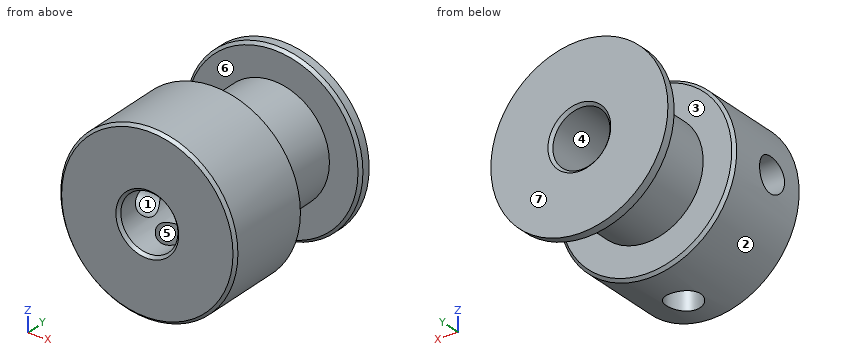
Autodesk Inventor part; units mm, degrees
ref_plane "YZ Plane" through (0, 0, 0) normal (1, 0, 0) x (0, 1, 0)
ref_plane "XZ Plane" through (0, 0, 0) normal (0, 1, 0) x (-1, 0, 0)
ref_plane "XY Plane" through (0, 0, 0) normal (0, 0, 1) x (1, 0, 0)
sketch "Эскиз1" plane through (0, 0, 0) normal (0, 1, 0) x (-1, 0, 0)
  circle A0 centre (0, 0) radius 7.75
  dimension "d0" = 15.5
extrude "Выдавливание1" add sketch "Эскиз1" along normal blind 8
sketch "Эскиз2" plane through (0, 8, 0) normal (0, 1, 0) x (1, 0, 0)
  circle A0 centre (0, 0) radius 5
  dimension "d3" = 10
extrude "Выдавливание2" add sketch "Эскиз2" along normal blind 7
sketch "Эскиз3" plane through (0, 15, 0) normal (0, 1, 0) x (1, 0, 0)
  circle A0 centre (0, 0) radius 7.75
extrude "Выдавливание3" add sketch "Эскиз3" along normal blind 1
chamfer "Фаска1" distance 0.25 angle 45 3 edges at (-7.75, 15, 0) (7.75, 8, 0) (7.75, 0, 0)
sketch "Эскиз4" plane through (0, 0, 0) normal (0, -1, 0) x (1, 0, 0)
  circle A0 centre (0, 0) radius 2.5
  dimension "d11" = 5
extrude "Выдавливание4" cut sketch "Эскиз4" against normal through all
chamfer "Фаска2" distance 0.25 angle 45 2 edges at (-2.5, 16, 0) (-2.5, 0, 0)
sketch "Эскиз5" plane through (0, 0, 0) normal (1, 0, 0) x (0, 1, 0)
  circle A0 centre (3.5, 0) radius 1.5
  point P0 (0, 0)
  dimension "d18" = 3
extrude "Выдавливание5" cut sketch "Эскиз5" against normal through all
sketch "Эскиз6" plane through (0, 0, 0) normal (0, 0, 1) x (1, 0, 0)
  circle A0 centre (0, 3.5) radius 1.5
  point P0 (0, 0)
  dimension "d22" = 3
extrude "Выдавливание6" cut sketch "Эскиз6" against normal through all
properties part number "GT2-20t"
Can you work these out from the model? Positions are in its coordinate system, mm. Face numbers are marked on the shaded views. A direction names the side the tool comes from. Coordinates: 2 decimals unless noted, no trailing zeros. Loops run counter-clockwise (first coordinate to the right, second up) from the corner with the lowest first, then second, coordinate; pieces in that order, holes last. Notation, with made-up numbers: (-29.75, 65) - (-6.75, 65) arc R36 ccw to (-6.75, 101) - close; hole circle Ø6 at (-14.75, 64). An arc over 180 degrees is marked (long way). Answer as a JSON object with one key per item and string values. Group by question number.
Item 1: If we mould it in two halves opening along Z, with no side actions, what happens to the marked faces 1, 2, 3 and 4? For each: released by +Z, released by -Z, zero draft, split by the parting line, or undercut.
Item 2: On a 3-axis mill with a long thin cutter (end or side, diameter ignored), from which of +Z, -Z, +X, -X, +Y, -Y can I reach the whole of each face in a straight line? I mean the marked faces 5, 6 and 7. Say none if no direction works.
Item 3: If I drill on L1, parallel to X at y = 12.5, z = 0; L2, parallel to Y at x = -3.5, z = 4.5; L3, parallel to Y at x = -6, z = -1.25, over which ranges is the centre line in solid material (lowest first)? Write a range as from..to.
Item 4: If we section it at D-D (y = 14.75): List the corners of the cut face in (x, z) for me, plus the area to 3 significant figures.
Item 5: If we section it at B-B (y = 4.5): List the corners of the cut face in (x, z) for me, plus the area to 3 significant figures.
Item 6: For pin 1 (4 mm diameter, centred on y = 10.5, z = -3, fed in from +X); pin 2 (1.8 mm diameter, centred on x = 0, y = 3.5, fed in from -Z); pin 3 (2 mm diameter, centred on x = -1, y = 13.5, fed in from +Z), each with a flat end and sliding along its axis, tell me the tip position at first contact or that it passes through.
Item 7: If we section it at A-A (z = 0): State how many separate pieces and enclosed holes the cut face has, plus the area to 3 significant figures.
Returned:
{
 "1": {"face 1": "undercut", "face 2": "split by the parting line", "face 3": "zero draft", "face 4": "undercut"},
 "2": {"face 5": "-Z", "face 6": "none", "face 7": "+Z, -Z, +X, -X, +Y"},
 "3": {"L1": "x = -5..-2.5, 2.5..5", "L2": "y = 0..8, 15..16", "L3": "y = 0..2.67, 4.33..8, 15..16"},
 "4": {"outline": "circle Ø10 at (0, 0); hole circle Ø5 at (0, 0)", "area": "58.9 mm²"},
 "5": {"outline": "(-7.67, -1.12) arc R7.75 ccw to (-1.12, -7.67) - (-1.12, -2.24) arc R2.5 cw to (-2.24, -1.12) - close; (-7.67, 1.12) - (-2.24, 1.12) arc R2.5 cw (long way) to (1.12, -2.24) - (1.12, -7.67) arc R7.75 ccw (long way) to start", "area": "145 mm²"},
 "6": {"pin 1": "stops at x = 4.9", "pin 2": "stops at z = 2.33", "pin 3": "stops at z = 5"},
 "7": {"separate pieces": "3", "enclosed holes": "0", "area": "113 mm²"}
}
